from build123d import *

# Parameters (mm, degrees)
BOSS_EXTRUDE1_DEPTH     = 3.175
F_1_4_CLEARANCE_HOLE1_D = 6.7564
F_10_CLEARANCE_HOLE1_D  = 5.1054
CUT_EXTRUDE1_DEPTH      = 93.539131925


with BuildPart() as part:
    # Sketch1 → Boss-Extrude1 (new body)
    with BuildSketch(Plane.XY):
        with BuildLine():
            Line((0, 58.7375), (63.5, 58.7375))
            ThreePointArc((63.5, 58.7375), (69.112660076, 56.412660076), (71.4375, 50.8))
            Line((71.4375, 50.8), (71.4375, 25.4))
            ThreePointArc((71.4375, 25.4), (70.072783642, 20.950008826), (66.447913494, 18.030216266))
            Line((66.447913494, 18.030216266), (2.947913494, -7.369783734))
            ThreePointArc((2.947913494, -7.369783734), (-4.449991174, -6.572783642), (-7.9375, 0))
            Line((-7.9375, 0), (-7.9375, 50.8))
            ThreePointArc((-7.9375, 50.8), (-5.612660076, 56.412660076), (0, 58.7375))
        make_face()
    extrude(amount=BOSS_EXTRUDE1_DEPTH)

    # 1/4 Clearance Hole1 (through all)
    with Locations(Plane.XY.offset(3.175)):
        with Locations((63.5, 50.8), (63.5, 25.4)):
            Hole(F_1_4_CLEARANCE_HOLE1_D / 2)

    # #10 Clearance Hole1 (through all)
    with Locations(Plane.XY.offset(3.175)):
        with Locations((0, 50.8), (0, 0)):
            Hole(F_10_CLEARANCE_HOLE1_D / 2)

    # Sketch6 → Cut-Extrude1 (cut, through all)
    with BuildSketch(Plane.XY.offset(3.175)):
        with BuildLine():
            Line((36.095363714, 32.942274862), (5.575352966, 45.150279161))
            ThreePointArc((5.575352966, 45.150279161), (2.259913756, 43.191012152), (-1.5875, 43.022870067))
            Line((-1.5875, 43.022870067), (-1.5875, 7.777129933))
            ThreePointArc((-1.5875, 7.777129933), (1.120121639, 7.858068068), (3.697288027, 7.023814312))
            Line((3.697288027, 7.023814312), (36.095363714, 32.942274862))
        make_face()
        with BuildLine():
            Line((7.933683761, 51.046106148), (41.794663135, 37.501714399))
            Line((41.794663135, 37.501714399), (55.835898421, 48.734702628))
            ThreePointArc((55.835898421, 48.734702628), (55.566297219, 50.554507771), (55.722870067, 52.3875))
            Line((55.722870067, 52.3875), (7.777129933, 52.3875))
            ThreePointArc((7.777129933, 52.3875), (7.883987005, 51.720138659), (7.933683761, 51.046106148))
        make_face()
        with BuildLine():
            Line((59.802711973, 43.776185688), (48.571302953, 34.791058471))
            Line((48.571302953, 34.791058471), (57.924647034, 31.049720839))
            ThreePointArc((57.924647034, 31.049720839), (61.240086244, 33.008987848), (65.0875, 33.177129933))
            Line((65.0875, 33.177129933), (65.0875, 43.022870067))
            ThreePointArc((65.0875, 43.022870067), (62.379878361, 42.941931932), (59.802711973, 43.776185688))
        make_face()
        with BuildLine():
            Line((55.566316239, 25.153893852), (42.872003532, 30.231618935))
            Line((42.872003532, 30.231618935), (7.664101579, 2.065297372))
            ThreePointArc((7.664101579, 2.065297372), (7.744125689, 1.741385529), (7.810466564, 1.414396799))
            Line((7.810466564, 1.414396799), (56.868698834, 21.037689707))
            ThreePointArc((56.868698834, 21.037689707), (55.932273748, 23.005542728), (55.566316239, 25.153893852))
        make_face()
    extrude(amount=-CUT_EXTRUDE1_DEPTH, mode=Mode.SUBTRACT)


solid = part.part
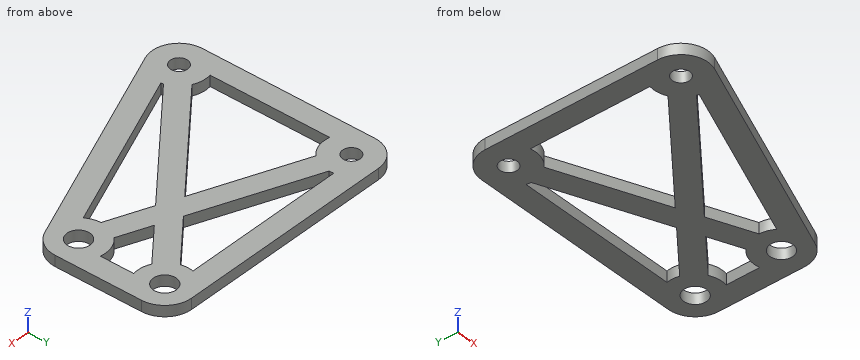
Design review of the part built by this model. Coordinates are the model's own, in mm. Round coordinates to 2 decimals unless told otherwise and drop trailing zeros. Write each loop counter-clockwise with the first axis right and the second up, starting at its lowest first coordinate (ties: lowest second). Pieces come first, ordered by that corner, then holes. Notation, with made-up numbers: (25.5, 8) -> (63.5, 8) arc R9 cw to (63.5, 17) -> close; hole circle Ø1 at (68.25, -39). An arc over 180 degrees is marked (long way). One line per item, written item: value. Start each with the question number.
Q1. Add section C-C (x = 32.5). Give the boundary of the cut face in (y, z) (1 decimal), then the cut area to 3 significant figures.
Q2. Add section D-D (x = 6.5). Give the boundary of the cut face in (y, z) (1 decimal), then the cut area to 3 significant figures.
Q3. To check wall thickness, follow probe 1 along Y at (x, z) = (0, 0.9); probe 2 along Y at (x, z) = (38.5, 2.1); probe 3 along Y at (x, z) = (33, 0.55). State the ranges of each line that lie inside material, in increasing order.
Q4. Add section B-B (y = 14). Give the boundary of the cut face in (x, z) (1 decimal), then the cut area to 3 significant figures.
Q5. Insertion check: P1, Ø5.5, axis at x = 63.5, y = 50.8, coming from the -Z side; P2, Ø1, axis at x = 20, z = 2, coming from the -Y side. Each pin has a flat end and moves straight along its axis. Give the tip position at first contact, or say it passes through.
Q6. Add section A-A (z = 1.8). State how many separate pieces and enclosed holes the cut face has, then the cut area to 3 significant figures.
Response:
1. outline: (4.5, 0) -> (11.3, 0) -> (11.3, 3.2) -> (4.5, 3.2) -> close; (21.9, 0) -> (30.1, 0) -> (30.1, 3.2) -> (21.9, 3.2) -> close; (34.4, 0) -> (41.2, 0) -> (41.2, 3.2) -> (34.4, 3.2) -> close; (52.4, 0) -> (58.7, 0) -> (58.7, 3.2) -> (52.4, 3.2) -> close
1. area: 89.4 mm^2
2. outline: (-5.9, 0) -> (9.3, 0) -> (9.3, 3.2) -> (-5.9, 3.2) -> close; (44.8, 0) -> (58.7, 0) -> (58.7, 3.2) -> (44.8, 3.2) -> close
2. area: 92.6 mm^2
3. probe 1: y = -7.94 to -2.55, 2.55 to 7.94, 42.86 to 48.25, 53.35 to 58.74
3. probe 2: y = 6.85 to 13.69, 26.73 to 38.82, 52.39 to 58.74
3. probe 3: y = 4.65 to 11.49, 22.33 to 30.47, 34.18 to 41.02, 52.39 to 58.74
4. outline: (-7.9, 0) -> (-1.6, 0) -> (-1.6, 3.2) -> (-7.9, 3.2) -> close; (12.4, 0) -> (22.6, 0) -> (22.6, 3.2) -> (12.4, 3.2) -> close; (39.3, 0) -> (56.4, 0) -> (56.4, 3.2) -> (39.3, 3.2) -> close
4. area: 107 mm^2
5. P1: passes through
5. P2: stops at y = -0.75
6. separate pieces: 1
6. enclosed holes: 8
6. area: 2,410 mm^2
